For this review, take the finished solid that the model builds, in its own axes (mm). Face numbers are marked on the shaded views. A direction names the side the tool comes from. Give positions to 0.01 mm unless a question says otherwise; leave off trailing zeros. Write each loop counter-clockwise with the first axis right and the second up, starting at its lowest first coordinate (ties: lowest second). Pieces come first, ordered by that corner, then holes. Notation, with made-up numbers: (-4, -33.75) -> (50, -33.75) arc R9 ccw to (50, -19.75) -> close; hole circle Ø8 at (-15, 89.25). An arc over 180 degrees is marked (long way). Answer as CSV lines item,"result".
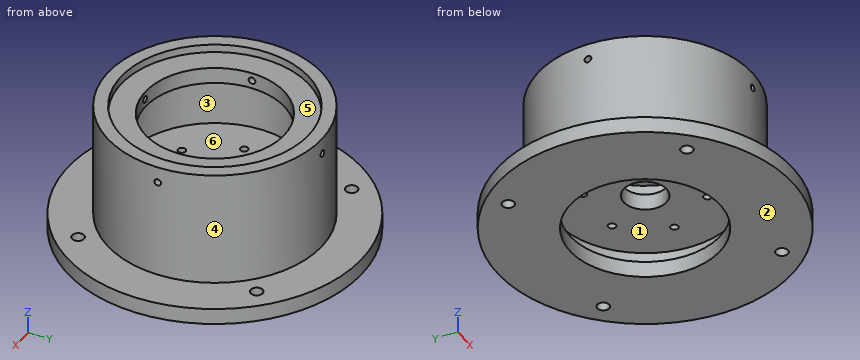
```python
from build123d import *

# Parameters (mm, degrees)
BRIDA_START                               = 10
SK_BRIDA_R                                = 55
BRIDA_DEPTH                               = 6
TUBO_START                                = 16
SK_TUBO_R                                 = 40
SK_TUBO_R_2                               = 33
TUBO_DEPTH                                = 34
ARO_RODAMIENTO_START                      = 50
SK_ARO_RODAMIENTO_R                       = 40
SK_ARO_RODAMIENTO_R_2                     = 26
ARO_RODAMIENTO_DEPTH                      = 6
ASIENTO_ARANDELA_ALOJAMIENTO_51110_START  = 56
SK_ASIENTO_ARANDELA_ALOJAMIENTO_51110_R   = 40
SK_ASIENTO_ARANDELA_ALOJAMIENTO_51110_R_2 = 35.1
ASIENTO_ARANDELA_ALOJAMIENTO_51110_DEPTH  = 3
PLACA_MOTOR_START                         = 23
SK_PLACA_MOTOR_R                          = 33
PLACA_MOTOR_DEPTH                         = 6
HUECO_BRIDA_START                         = 10
SK_HUECO_BRIDA_R                          = 28
HUECO_BRIDA_DEPTH                         = 13
CENTRO_MOTOR_START                        = 23
SK_CENTRO_MOTOR_R                         = 8
CENTRO_MOTOR_DEPTH                        = 6
PASANTES_M2_5_MOTOR_START                 = 23
SK_PASANTES_M2_5_MOTOR_R                  = 1.45
PASANTES_M2_5_MOTOR_DEPTH                 = 6
PASANTES_M4_BRIDA_START                   = 10
SK_PASANTES_M4_BRIDA_R                    = 2.25
PASANTES_M4_BRIDA_DEPTH                   = 6
ROSCA_M3_CUBIERTA_A_DEPTH                 = 98.626840572
ROSCA_M3_CUBIERTA_A_DEPTH_BACK            = 98.626840572
CROQUIS1_R                                = 1.25
ROSCA_M3_CUBIERTA_B_DEPTH                 = 98.626840632
ROSCA_M3_CUBIERTA_B_DEPTH_BACK            = 98.626840632
CROQUIS2_R                                = 1.25


with BuildPart() as part:
    # Sk_Brida → Brida (new body)
    with BuildSketch(Plane.XY.offset(BRIDA_START)):
        Circle(SK_BRIDA_R)
    extrude(amount=BRIDA_DEPTH)

    # Sk_Tubo → Tubo (add)
    with BuildSketch(Plane.XY.offset(TUBO_START)):
        Circle(SK_TUBO_R)
        Circle(SK_TUBO_R_2, mode=Mode.SUBTRACT)
    extrude(amount=TUBO_DEPTH)

    # Sk_Aro_rodamiento → Aro_rodamiento (add)
    with BuildSketch(Plane.XY.offset(ARO_RODAMIENTO_START)):
        Circle(SK_ARO_RODAMIENTO_R)
        Circle(SK_ARO_RODAMIENTO_R_2, mode=Mode.SUBTRACT)
    extrude(amount=ARO_RODAMIENTO_DEPTH)

    # Sk_Asiento_arandela_alojamiento_51110 → Asiento_arandela_alojamiento_51110 (add)
    with BuildSketch(Plane.XY.offset(ASIENTO_ARANDELA_ALOJAMIENTO_51110_START)):
        Circle(SK_ASIENTO_ARANDELA_ALOJAMIENTO_51110_R)
        Circle(SK_ASIENTO_ARANDELA_ALOJAMIENTO_51110_R_2, mode=Mode.SUBTRACT)
    extrude(amount=ASIENTO_ARANDELA_ALOJAMIENTO_51110_DEPTH)

    # Sk_Placa_motor → Placa_motor (add)
    with BuildSketch(Plane.XY.offset(PLACA_MOTOR_START)):
        Circle(SK_PLACA_MOTOR_R)
    extrude(amount=PLACA_MOTOR_DEPTH)

    # Sk_Hueco_brida → Hueco_brida (cut)
    with BuildSketch(Plane.XY.offset(HUECO_BRIDA_START)):
        Circle(SK_HUECO_BRIDA_R)
    extrude(amount=HUECO_BRIDA_DEPTH, mode=Mode.SUBTRACT)

    # Sk_Centro_motor → Centro_motor (cut)
    with BuildSketch(Plane.XY.offset(CENTRO_MOTOR_START)):
        Circle(SK_CENTRO_MOTOR_R)
    extrude(amount=CENTRO_MOTOR_DEPTH, mode=Mode.SUBTRACT)

    # Sk_Pasantes_M2-5_motor → Pasantes_M2-5_motor (cut)
    with BuildSketch(Plane.XY.offset(PASANTES_M2_5_MOTOR_START)):
        with Locations((20.5, 0)):
            Circle(SK_PASANTES_M2_5_MOTOR_R)
        with Locations((10.25, 17.753520778)):
            Circle(SK_PASANTES_M2_5_MOTOR_R)
        with Locations((-10.25, 17.753520778)):
            Circle(SK_PASANTES_M2_5_MOTOR_R)
        with Locations((-20.5, 0)):
            Circle(SK_PASANTES_M2_5_MOTOR_R)
        with Locations((-10.25, -17.753520778)):
            Circle(SK_PASANTES_M2_5_MOTOR_R)
        with Locations((10.25, -17.753520778)):
            Circle(SK_PASANTES_M2_5_MOTOR_R)
    extrude(amount=PASANTES_M2_5_MOTOR_DEPTH, mode=Mode.SUBTRACT)

    # Sk_Pasantes_M4_brida → Pasantes_M4_brida (cut)
    with BuildSketch(Plane.XY.offset(PASANTES_M4_BRIDA_START)):
        with Locations((33.234018716, 33.234018716)):
            Circle(SK_PASANTES_M4_BRIDA_R)
        with Locations((-33.234018716, 33.234018716)):
            Circle(SK_PASANTES_M4_BRIDA_R)
        with Locations((-33.234018716, -33.234018716)):
            Circle(SK_PASANTES_M4_BRIDA_R)
        with Locations((33.234018716, -33.234018716)):
            Circle(SK_PASANTES_M4_BRIDA_R)
    extrude(amount=PASANTES_M4_BRIDA_DEPTH, mode=Mode.SUBTRACT)

    # Croquis1 → Rosca_M3_cubierta_A (cut, two sides: drawn at the far end of the back side and taken through both)
    with BuildSketch(Plane(origin=(0, 0, 0), x_dir=(1, 0, 0), z_dir=(0, 1, 0)).offset(-ROSCA_M3_CUBIERTA_A_DEPTH_BACK)):
        with Locations(Location((0, -53, 0), (0, 0, 270))):
            Circle(CROQUIS1_R)
    extrude(amount=ROSCA_M3_CUBIERTA_A_DEPTH + ROSCA_M3_CUBIERTA_A_DEPTH_BACK, mode=Mode.SUBTRACT)

    # Croquis2 → Rosca_M3_cubierta_B (cut, two sides: drawn at the far end of the back side and taken through both)
    with BuildSketch(Plane(origin=(0, 0, 0), x_dir=(0, 0, -1), z_dir=(1, 0, 0)).offset(-ROSCA_M3_CUBIERTA_B_DEPTH_BACK)):
        with Locations((-53, 0)):
            Circle(CROQUIS2_R)
    extrude(amount=ROSCA_M3_CUBIERTA_B_DEPTH + ROSCA_M3_CUBIERTA_B_DEPTH_BACK, mode=Mode.SUBTRACT)


solid = part.part
```
Q1. Draft analysis for pull direction X (two halves, no side actions). For the marked faces 1, 2, 3 and 4, state which applies: released by +X, released by -X, zero draft, split by the parting line, or undercut.
Answer block:
face 1,"undercut"
face 2,"zero draft"
face 3,"undercut"
face 4,"split by the parting line"
Q2. To check wall thickness, follow probe 1 along Z at (x, y) = (-8, -28); probe 2 along Z at (x, y) = (0, -32.75); probe 3 along Z at (x, y) = (0, -35.5). State the ranges of each line that lie inside material, in increasing order. Write a range as [from, to].
Answer block:
probe 1,"z = [10, 16], [23, 29], [50, 56]"
probe 2,"z = [10, 16], [23, 29], [50, 51.75], [54.25, 56]"
probe 3,"z = [10, 51.75], [54.25, 59]"
Q3. For the marked faces 5 and 6, list the 3-axis set-ups (+Z, -Z, +X, -X, +Y, -Y) from which the entire face can be reached by the end or side of a thin tool; tool diameter is ignored.
Answer block:
face 5,"+Z"
face 6,"none"
Q4. Clearance check with flat-ended pins moving along their axes: pin 1 (2 mm diameter, centred on x = -16.5, z = 18.5, fed in from -Y); pin 2 (4.5 mm diameter, centred on x = 10.25, y = 17.75, fed in from -Z); pin 3 (20 mm diameter, centred on x = 5.5, y = 7.5, fed in from +Z). State where each tip first meets the part, or that it passes through.
Answer block:
pin 1,"stops at y = -36.87"
pin 2,"stops at z = 23"
pin 3,"stops at z = 29"
Q5. Add section C-C (y = 24). Write out the cut boundary in (x, z), plus the area to 3 significant figures.
Answer block:
outline,"(-49.49, 10) -> (-14.42, 10) -> (-14.42, 16) -> (-22.65, 16) -> (-22.65, 23) -> (22.65, 23) -> (22.65, 16) -> (14.42, 16) -> (14.42, 10) -> (49.49, 10) -> (49.49, 16) -> (32, 16) -> (32, 59) -> (25.61, 59) -> (25.61, 56) -> (10, 56) -> (10, 50) -> (22.65, 50) -> (22.65, 29) -> (-22.65, 29) -> (-22.65, 50) -> (-10, 50) -> (-10, 56) -> (-25.61, 56) -> (-25.61, 59) -> (-32, 59) -> (-32, 16) -> (-49.49, 16) -> close"
area,"1,630 mm2"
Q6. Add section B-B (z = 31). Write out the cut boundary in (x, y), plus the area to 3 significant figures.
Answer block:
outline,"circle Ø80 at (0, 0); hole circle Ø66 at (0, 0)"
area,"1,610 mm2"
Q7. Add section D-D (x = -10.25). State how many separate pieces and enclosed holes the cut face has, plus the area to 3 significant figures.
Answer block:
separate pieces,"3"
enclosed holes,"0"
area,"1,380 mm2"
